Read the model definition and answer for the solid it produces. Units are mm, in the model's axes. A direction names the side the tool comes from. Round coordinates to 2 decimals unless told otherwise and drop trailing zeros. Write each loop counter-clockwise with the first axis right and the second up, starting at its lowest first coordinate (ties: lowest second). Pieces come first, ordered by that corner, then holes. Notation, with made-up numbers: (-24, 19.5) - (7, 19.5) arc R19 ccw to (7, 51.5) - close; hole circle Ø4 at (-26.75, 85). An arc over 180 degrees is marked (long way). One line per item, written item: value. Start each with the question number.
(1) The mould has two halves that part along Y. Classify faces 1 (the face through (8.023, 0.07, 0.74)), 2 (the face through (4.124, 0.04, 0.456)), 3 (the face through (-0.3, 2.48, 0.74)): +Y half, -Y half, draft (parallel to the pull), parting line (faces both ways), or undercut.
(2) A cutting plane is placed at D-D, the plane y = -0.65. Determine the outline of the cut face in (x, z), plus the area to 3 significant figures.
(3) A cutting plane is placed at A-A, the plane y = 0. Determine the outline of the cut face in (x, z).
(4) For faces 4 (the face through (3.075, 0.086, 2.218)), 5 (the face through (-6.976, -0.041, 0.74)), determine the directions among +Z, -Z, +X, -X, +Y, -Y from which every point of the face is accessible in a straight line to the end or side of a thin tool.
(5) A cutting plane is placed at B-B, the plane z = 0.7. Determine the outline of the cut face in (x, y), plus the area to 3 significant figures.
(6) Find the intervals of material crossed by L1, parallel to X at y = -0.05, z = 2.85; L2, parallel to Z at x = -1.75, y = 0.3; L3, parallel to X at y = -1.65, z = 2, in increasing order.
(7) A cutting plane is placed at C-C, the plane x = 2.75. Determine the outline of the cut face in (y, z), plus the area to 3 significant figures.
(8) Flat-ended cylindrical pins translate along their axes: pin 1 Ø2 at (x, y) = (-3, 1.5) entering from +Z; pin 2 Ø3 at (x, y) = (5.02, 0) entering from -Z; pin 3 Ø1.5 at (y, z) = (1, 1.5) entering from +X. Find the tip coordinate at first contact, or state that the pin passes through.
from build123d import *

# Parameters (mm, degrees)
EXTRUSION1_DEPTH = 1.5
ESQUISSE2_R      = 2.925
EXTRUSION2_DEPTH = 2
ESQUISSE3_R      = 0.9
EXTRUSION3_DEPTH = 10.253328027
ESQUISSE4_R      = 1.95
EXTRUSION4_DEPTH = 2.6


with BuildPart() as part:
    # Esquisse1 → Extrusion1 (new body)
    with BuildSketch(Plane.XY):
        with BuildLine():
            Line((-5.176654091, 1.989974874), (4.723345909, 2.984962311))
            ThreePointArc((4.723345909, 2.984962311), (8.023345909, 0), (4.723345909, -2.984962311))
            Line((4.723345909, -2.984962311), (-5.176654091, -1.989974874))
            ThreePointArc((-5.176654091, -1.989974874), (-6.976654091, 0), (-5.176654091, 1.989974874))
        make_face()
    extrude(amount=EXTRUSION1_DEPTH)

    # Esquisse2 → Extrusion2 (add)
    with BuildSketch(Plane.XY.offset(1.5)):
        with Locations((5.023345909, 0)):
            Circle(ESQUISSE2_R)
    extrude(amount=EXTRUSION2_DEPTH)

    # Esquisse3 → Extrusion3 (cut, through all)
    with BuildSketch(Plane.XY.offset(3.5)):
        with Locations((5.023345909, 0)):
            Circle(ESQUISSE3_R)
    extrude(amount=-EXTRUSION3_DEPTH, mode=Mode.SUBTRACT)

    # Esquisse4 → Extrusion4 (cut)
    with BuildSketch(Plane.XY.offset(3.5)):
        with Locations((5.023345909, 0)):
            Circle(ESQUISSE4_R)
    extrude(amount=-EXTRUSION4_DEPTH, mode=Mode.SUBTRACT)


solid = part.part
Here are the results:
1. face 1: parting line
1. face 2: undercut
1. face 3: +Y half
2. outline: (-6.87, 0) - (4.4, 0) - (4.4, 0.9) - (3.18, 0.9) - (3.18, 3.5) - (2.17, 3.5) - (2.17, 1.5) - (-6.87, 1.5) - close; (5.65, 0) - (7.95, 0) - (7.95, 1.5) - (7.88, 1.5) - (7.88, 3.5) - (6.86, 3.5) - (6.86, 0.9) - (5.65, 0.9) - close
2. area: 23.0 mm²
3. outline: (-6.98, 0) - (4.12, 0) - (4.12, 0.9) - (3.07, 0.9) - (3.07, 3.5) - (2.1, 3.5) - (2.1, 1.5) - (-6.98, 1.5) - close; (5.92, 0) - (8.02, 0) - (8.02, 1.5) - (7.95, 1.5) - (7.95, 3.5) - (6.97, 3.5) - (6.97, 0.9) - (5.92, 0.9) - close
4. face 4: +Z
4. face 5: +Z, -Z, -X
5. outline: (-5.18, -1.99) - (4.72, -2.98) arc R3 ccw (long way) to (4.72, 2.98) - (-5.18, 1.99) arc R2 ccw to start; hole circle Ø1.8 at (5.02, 0)
5. area: 68.1 mm²
6. L1: 2.1 to 3.07, 6.97 to 7.95
6. L2: 0 to 1.5
6. L3: 2.61 to 3.98, 6.06 to 7.44
7. outline: (-2.79, 0) - (2.79, 0) - (2.79, 1.5) - (1.84, 1.5) - (1.84, 3.5) - (-1.84, 3.5) - (-1.84, 1.5) - (-2.79, 1.5) - close
7. area: 15.7 mm²
8. pin 1: z = 1.5
8. pin 2: z = 0
8. pin 3: x = 8.01
